from build123d import *

# Parameters (mm, degrees)
F1_DEPTH = 4
F2_DEPTH = 2
F3_DEPTH = 4


# Not quite as in the source:
# - a feature names something its author has since deleted; it is built from what else it names


with BuildPart() as f1:
    # F0 (on Top) → F1 (new body, symmetric)
    with BuildSketch(Plane.XY):
        with BuildLine():
            Line((55, 40), (55, 55))
            Line((55, 55), (40, 55))
            ThreePointArc((40, 55), (21.3600093633, 43.8733083646), (0, 40))
            Line((0, 40), (0, 37.5))
            Line((0, 37.5), (12.5, 37.5))
            Line((12.5, 37.5), (12.5, 0))
            Line((12.5, 0), (21, 0))
            Line((21, 0), (21, 16))
            Line((21, 16), (32, 16))
            Line((32, 16), (32, 0))
            Line((32, 0), (40, 0))
            ThreePointArc((40, 0), (43.8733083645, 21.3600093633), (55, 40))
        make_face()
        with BuildLine():
            ThreePointArc((35.5367965644, 33.7867965644), (32.1700073825, 33.1171005578), (35.0242334315, 35.0242334315))
            ThreePointArc((35.0242334315, 35.0242334315), (35.4035857463, 34.456492571), (35.5367965644, 33.7867965644))
        make_face(mode=Mode.SUBTRACT)
        with BuildLine():
            ThreePointArc((46.6914953211, 46.6914953211), (46.6914953211, 49.1663690552), (49.1663690552, 49.1663690552))
            ThreePointArc((49.1663690552, 49.1663690552), (49.54572137, 48.5986281948), (49.6789321881, 47.9289321881))
            ThreePointArc((49.6789321881, 47.9289321881), (48.5986281948, 46.3121430062), (46.6914953211, 46.6914953211))
        make_face(mode=Mode.SUBTRACT)
        with BuildLine():
            Line((-12.5, -37.5), (-12.5, 0))
            Line((-12.5, 0), (-13.6673537509, 0))
            ThreePointArc((-13.6673537509, 0), (-15.1673537509, -1.5), (-16.6673537509, 0))
            Line((-16.6673537509, 0), (-21, 0))
            Line((-21, 0), (-21, -16))
            Line((-21, -16), (-32, -16))
            Line((-32, -16), (-32, 0))
            Line((-32, 0), (-36.7343537509, 0))
            Line((-36.7343537509, 0), (-40, 0))
            ThreePointArc((-40, 0), (-43.8733083645, -21.3600093633), (-55, -40))
            Line((-55, -40), (-55, -55))
            Line((-55, -55), (-40, -55))
            ThreePointArc((-40, -55), (-21.3600093633, -43.8733083646), (0, -40))
            Line((0, -40), (0, -37.5))
            Line((0, -37.5), (-12.5, -37.5))
        make_face()
        with BuildLine():
            ThreePointArc((-46.1789321881, -47.9289321881), (-47.2592361815, -49.54572137), (-49.1663690552, -49.1663690552))
            ThreePointArc((-49.1663690552, -49.1663690552), (-49.1663690552, -46.6914953211), (-46.6914953211, -46.6914953211))
            ThreePointArc((-46.6914953211, -46.6914953211), (-46.3121430062, -47.2592361815), (-46.1789321881, -47.9289321881))
        make_face(mode=Mode.SUBTRACT)
        with BuildLine():
            ThreePointArc((-32.0367965644, -33.7867965644), (-33.1171005578, -35.4035857463), (-35.0242334315, -35.0242334315))
            ThreePointArc((-35.0242334315, -35.0242334315), (-34.456492571, -32.1700073825), (-32.0367965644, -33.7867965644))
        make_face(mode=Mode.SUBTRACT)
        with BuildLine():
            ThreePointArc((-35.2343537509, -21.567), (-37.7950139227, -22.6276601718), (-36.7343537509, -20.067))
            ThreePointArc((-36.7343537509, -20.067), (-35.6736935792, -20.5063398282), (-35.2343537509, -21.567))
        make_face(mode=Mode.SUBTRACT)
        with BuildLine():
            Line((0, 37.5), (0, 40))
            ThreePointArc((0, 40), (-21.3600093633, 43.8733083645), (-40, 55))
            Line((-40, 55), (-55, 55))
            Line((-55, 55), (-55, 40))
            ThreePointArc((-55, 40), (-43.8733083646, 21.3600093633), (-40, 0))
            Line((-40, 0), (-36.7343537509, 0))
            Line((-36.7343537509, 0), (-32, 0))
            Line((-32, 0), (-32, 16))
            Line((-32, 16), (-21, 16))
            Line((-21, 16), (-21, 0))
            Line((-21, 0), (-16.6673537509, 0))
            ThreePointArc((-16.6673537509, 0), (-15.1673537509, 1.5), (-13.6673537509, 0))
            Line((-13.6673537509, 0), (-12.5, 0))
            Line((-12.5, 0), (-12.5, 37.5))
            Line((-12.5, 37.5), (0, 37.5))
        make_face()
        with BuildLine():
            ThreePointArc((-35.2343537509, 21.567), (-35.6736935792, 20.5063398282), (-36.7343537509, 20.067))
            ThreePointArc((-36.7343537509, 20.067), (-37.7950139227, 22.6276601718), (-35.2343537509, 21.567))
        make_face(mode=Mode.SUBTRACT)
        with BuildLine():
            ThreePointArc((-32.0367965644, 33.7867965644), (-34.456492571, 32.1700073825), (-35.0242334315, 35.0242334315))
            ThreePointArc((-35.0242334315, 35.0242334315), (-33.1171005578, 35.4035857463), (-32.0367965644, 33.7867965644))
        make_face(mode=Mode.SUBTRACT)
        with BuildLine():
            ThreePointArc((-46.6914953211, 46.6914953211), (-49.1663690552, 46.6914953211), (-49.1663690552, 49.1663690552))
            ThreePointArc((-49.1663690552, 49.1663690552), (-47.2592361815, 49.54572137), (-46.1789321881, 47.9289321881))
            ThreePointArc((-46.1789321881, 47.9289321881), (-46.3121430062, 47.2592361815), (-46.6914953211, 46.6914953211))
        make_face(mode=Mode.SUBTRACT)
        with BuildLine():
            ThreePointArc((55, -40), (43.8733083646, -21.3600093633), (40, 0))
            Line((40, 0), (32, 0))
            Line((32, 0), (32, -16))
            Line((32, -16), (21, -16))
            Line((21, -16), (21, 0))
            Line((21, 0), (12.5, 0))
            Line((12.5, 0), (12.5, -37.5))
            Line((12.5, -37.5), (0, -37.5))
            Line((0, -37.5), (0, -40))
            ThreePointArc((0, -40), (21.3600093633, -43.8733083645), (40, -55))
            Line((40, -55), (55, -55))
            Line((55, -55), (55, -40))
        make_face()
        with BuildLine():
            ThreePointArc((49.6789321881, -47.9289321881), (49.54572137, -48.5986281948), (49.1663690552, -49.1663690552))
            ThreePointArc((49.1663690552, -49.1663690552), (46.6914953211, -49.1663690552), (46.6914953211, -46.6914953211))
            ThreePointArc((46.6914953211, -46.6914953211), (48.5986281948, -46.3121430062), (49.6789321881, -47.9289321881))
        make_face(mode=Mode.SUBTRACT)
        with BuildLine():
            ThreePointArc((35.5367965644, -33.7867965644), (35.4035857463, -34.456492571), (35.0242334315, -35.0242334315))
            ThreePointArc((35.0242334315, -35.0242334315), (32.1700073825, -33.1171005578), (35.5367965644, -33.7867965644))
        make_face(mode=Mode.SUBTRACT)
    extrude(amount=F1_DEPTH, both=True)

    # F0 (on Top) → F2 (join, symmetric)
    with BuildSketch(Plane.XY):
        Polygon((-4.8118475825, 0), (-12.5, 0), (-12.5, -37.5), (0, -37.5), (0, -23.5897935927), (-4.8118475825, -23.5897935927), align=None)
        Polygon((12.5, -37.5), (12.5, 0), (4.8118475825, 0), (4.8118475825, -23.5897935927), (0, -23.5897935927), (0, -37.5), align=None)
        Polygon((0, 23.5897935927), (0, 37.5), (-12.5, 37.5), (-12.5, 0), (-4.8118475825, 0), (-4.8118475825, 23.5897935927), align=None)
        Polygon((12.5, 37.5), (0, 37.5), (0, 23.5897935927), (4.8118475825, 23.5897935927), (4.8118475825, 0), (12.5, 0), align=None)
    extrude(amount=F2_DEPTH, both=True)

    # F0 (on Top) → F3 (join)
    with BuildSketch(Plane.XY):
        Polygon((-4.8118475825, 0), (-12.5, 0), (-12.5, -37.5), (0, -37.5), (0, -23.5897935927), (-4.8118475825, -23.5897935927), align=None)
        Polygon((12.5, -37.5), (12.5, 0), (4.8118475825, 0), (4.8118475825, -23.5897935927), (0, -23.5897935927), (0, -37.5), align=None)
        Polygon((0, 23.5897935927), (0, 37.5), (-12.5, 37.5), (-12.5, 0), (-4.8118475825, 0), (-4.8118475825, 23.5897935927), align=None)
        Polygon((12.5, 37.5), (0, 37.5), (0, 23.5897935927), (4.8118475825, 23.5897935927), (4.8118475825, 0), (12.5, 0), align=None)
    extrude(amount=-F3_DEPTH)


solid = f1.part
Input: part model. Units: mm. Frame: model coordinates. A direction names the side the tool comes from. Give positions to 0.01 mm unless a question says otherwise; leave off trailing zeros. Order: outer loops, then holes, each group sorted by start corner. A loop starts at its lowest first (then second) coordinate and runs counter-clockwise, first axis right, second up. Notation, with made-up numbers: M 30.25,3 L 88.25,3 A25 ccw 88.25,31 Z; hole C 47.25,14.25 d5. An arc over 180 degrees is marked long. Answer as a JSON object with one key per item and string values.
1. First-contact query: P1, Ø2, axis at y = 32.5, z = 2.5, coming from the -X side; P2, Ø4.5, axis at y = 4, z = -2, coming from the -X side; P3, Ø4, axis at y = -29, z = 2.5, coming from the +X side. Flat tips, straight axial feed; report the tip coordinate or a pass-through.
Result sheet:
{"P1": "x = -50.05", "P2": "x = -40.32", "P3": "x = 48.49"}
2. Cut plane C-C, the plane y = 18. Output: boundary loops of the cut face in (x, z).
Result sheet:
{"outline": "M -42.72,-4 L -4.81,-4 L -4.81,2 L -12.5,2 L -12.5,4 L -42.72,4 Z; M 4.81,-4 L 42.72,-4 L 42.72,4 L 12.5,4 L 12.5,2 L 4.81,2 Z"}
3. Ray query, line 1 (X direction, y = 21, z = 0); line 2 (X direction, y = -7.5, z = 0.5); line 3 (X direction, y = 4.5, z = -1.75). Return the intervals inside material, ascending. Write a range as [from, to].
Result sheet:
{"line 1": "[-43.74, -38.12], [-35.35, -4.81], [4.81, 43.74]", "line 2": "[-40.46, -32], [-21, -4.81], [4.81, 21], [32, 40.46]", "line 3": "[-40.17, -32], [-21, -4.81], [4.81, 21], [32, 40.17]"}
4. Cut plane A-A, the plane x = -43. Output: boundary loops of the cut face in (y, z).
Result sheet:
{"outline": "M -55,-4 L -18.87,-4 L -18.87,4 L -55,4 Z; M 18.87,-4 L 55,-4 L 55,4 L 18.87,4 Z"}
5. Cut plane D-D, the plane y = 29. Output: boundary loops of the cut face in (x, z), and give its area (3 significant figures).
Result sheet:
{"outline": "M -47.36,-4 L 47.36,-4 L 47.36,4 L 12.5,4 L 12.5,2 L -12.5,2 L -12.5,4 L -47.36,4 Z", "area": "708 mm²"}
6. Pull-direction query (X, two-part tool) for faces 1 (the cylindrical face through (-40.003, 0.611, 0.056)), 2 (the cylindrical face through (0.611, 40.003, 0.056)), 3 (the flat face through (55, 47, 0)), 4 (the flat face through (-47, 55, 0)); classes: +X half, -X half, draft (parallel to the pull), parting line (faces both ways), or undercut.
Result sheet:
{"face 1": "-X half", "face 2": "undercut", "face 3": "+X half", "face 4": "draft"}
7. Reachability of faces 5 (the flat face through (-13, 1, -4)), 6 (the flat face through (-4.812, 0, -1)), 7 (the flat face through (-6, 1, 2)) from +Z, -Z, +X, -X, +Y, -Y: full face, straight path, thin tool, end or side. Return the list, or none.
Result sheet:
{"face 5": "-Z, +X, -X, +Y, -Y", "face 6": "+Z, -Z", "face 7": "+Z"}
8. Cut plane B-B, the plane y = 0. Output: boundary loops of the cut face in (x, z).
Result sheet:
{"outline": "M -40,-4 L -32,-4 L -32,4 L -40,4 Z; M -21,-4 L -16.67,-4 L -16.67,4 L -21,4 Z; M -13.67,-4 L -4.81,-4 L -4.81,2 L -12.5,2 L -12.5,4 L -13.67,4 Z; M 4.81,-4 L 21,-4 L 21,4 L 12.5,4 L 12.5,2 L 4.81,2 Z; M 32,-4 L 40,-4 L 40,4 L 32,4 Z"}
